Check sheet for the modelled part. Datum: model origin and axes. Units: mm. Round coordinates to 2 decimals unless told otherwise and drop trailing zeros. Order: outer loops, then holes, each group sorted by start corner. A loop starts at its lowest first (then second) coordinate and runs counter-clockwise, first axis right, second up. Notation, with made-up numbers: (71.5, -26.5) -> (78.5, -26.5) arc R26 ccw to (78.5, -5.5) -> close; hole circle Ø1 at (47, -30.5). An arc over 180 degrees is marked (long way). Answer in a Markdown table with one row per item. Add a question column.
1. Sectioned sample at A-A, the plane x = 26. Record the boundary of the cut face in (y, z).
2. Depth check by flat-ended pin: P1, Ø1.2, axis at x = 129.5, z = -33, coming from the +Y side; P2, Ø1.2, axis at x = -1.5, y = 2, coming from the -Z side; P3, Ø3, axis at x = 129, z = -32.5, coming from the -Y side. Enter the tip coordinate at first touch or a pass-through.
3. Sectioned sample at B-B, the plane z = -7.5. Record the boundary of the cut face in (x, y) (3 decimals), then the cut area to 3 significant figures.
4. Material ranges on L1, parallel to Z at x = 51.5, y = 3.5; L2, parallel to Z at x = 86.5, y = 4; L3, parallel to Y at x = 65.5, z = -18.5, recorded low to high. Write a range as from..to.
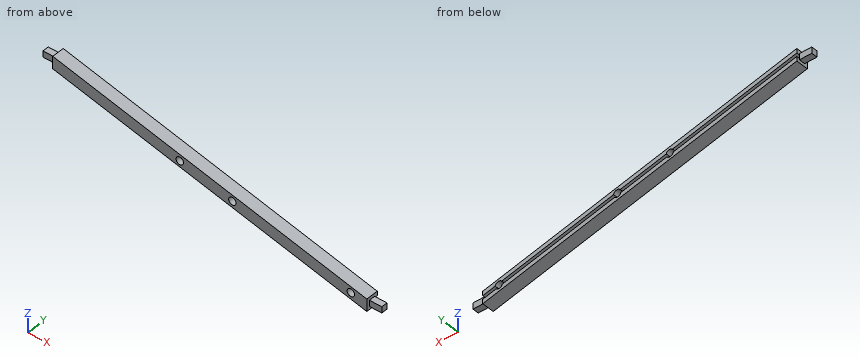
```python
from build123d import *

# Parameters (mm, degrees)
BOSS_EXTRUDE1_DEPTH = 5
SKETCH2_W           = 2.5
SKETCH2_H           = 2.5
BOSS_EXTRUDE2_DEPTH = 5
SKETCH3_W           = 2.5
SKETCH3_H           = 2.5
BOSS_EXTRUDE3_DEPTH = 5
SKETCH6_R           = 1.5
CUT_EXTRUDE1_DEPTH  = 5
CUT_EXTRUDE3_DEPTH  = 2


with BuildPart() as part:
    # Sketch1 → Boss-Extrude1 (new body)
    with BuildSketch(Plane(origin=(0, 0, 0), x_dir=(1, 0, 0), z_dir=(0, 1, 0))):
        Polygon((0, 5), (0, 0), (127.3, 30), (127.3, 35), align=None)
    extrude(amount=BOSS_EXTRUDE1_DEPTH)

    # Sketch2 → Boss-Extrude2 (add)
    with BuildSketch(Plane(origin=(127.3, 0, 0), x_dir=(0, 0, -1), z_dir=(1, 0, 0))):
        with Locations((32.5, 2.5)):
            Rectangle(SKETCH2_W, SKETCH2_H)
    extrude(amount=BOSS_EXTRUDE2_DEPTH)

    # Sketch3 → Boss-Extrude3 (add)
    with BuildSketch(Plane.ZY):
        with Locations((-2.5, 2.5)):
            Rectangle(SKETCH3_W, SKETCH3_H)
    extrude(amount=BOSS_EXTRUDE3_DEPTH)

    # Sketch6 → Cut-Extrude1 (cut)
    with BuildSketch(Plane.XZ):
        with Locations(Location((51.5, -14.705168766, 0), (0, 0, 270))):
            Circle(SKETCH6_R)
        with Locations(Location((72.8, -19.587839875, 0), (0, 0, 270))):
            Circle(SKETCH6_R)
        with Locations(Location((120.8, -30.899701619, 0), (0, 0, 270))):
            Circle(SKETCH6_R)
    extrude(amount=-CUT_EXTRUDE1_DEPTH, mode=Mode.SUBTRACT)

    # Sketch10 → Cut-Extrude3 (cut)
    with BuildSketch(Plane(origin=(0, 5, 0), x_dir=(1, 0, 0), z_dir=(0, 1, 0))):
        Polygon((0, 3.202061361), (0, 1.797938639), (127.3, 31.797938639), (127.3, 33.202061361), align=None)
    extrude(amount=-CUT_EXTRUDE3_DEPTH, mode=Mode.SUBTRACT)


solid = part.part
```
Answer key:
| question | item | result |
|---|---|---|
| 1 | outline | (0, -11.13) -> (5, -11.13) -> (5, -9.33) -> (3, -9.33) -> (3, -7.93) -> (5, -7.93) -> (5, -6.13) -> (0, -6.13) -> close |
| 2 | P1 | stops at y = 3.75 |
| 2 | P2 | stops at z = -3.75 |
| 2 | P3 | stops at y = 1.25 |
| 3 | outline | (10.608, 0) -> (31.825, 0) -> (31.825, 5) -> (24.196, 5) -> (24.196, 3) -> (18.238, 3) -> (18.238, 5) -> (10.608, 5) -> close |
| 3 | area | 94.2 mm² |
| 4 | L1 | z = -17.14..-16.21, -13.21..-12.14 |
| 4 | L2 | z = -25.38..-23.59, -22.18..-20.38 |
| 4 | L3 | y = 0..3 |
